from build123d import *

# Parameters (mm, degrees)
F0_W     = 130
F0_H     = 48
F1_DEPTH = 25
F3_DEPTH = 25.001
F4_R     = 1.5
F5_DEPTH = 25.001
F6_W     = 90
F6_H     = 48
F7_DEPTH = 5
F8_DEPTH = 25


with BuildPart() as f1:
    # F0 (on Top) → F1 (new body)
    with BuildSketch(Plane.XY):
        Rectangle(F0_W, F0_H)
    extrude(amount=F1_DEPTH)

    # F2 (on face) → F3 (cut, through all)
    with BuildSketch(Plane.XY.offset(25)):
        Polygon((7, -24), (0, -17), (-7, -24), align=None)
    extrude(amount=-F3_DEPTH, mode=Mode.SUBTRACT)

    # F4 (on face) → F5 (cut, through all)
    with BuildSketch(Plane.XY.offset(25)):
        with Locations((-55, 12)):
            Circle(F4_R)
        with Locations((-55, 2)):
            Circle(F4_R)
        with Locations((-55, -8)):
            Circle(F4_R)
        with Locations((55, 12)):
            Circle(F4_R)
        with Locations((55, 2)):
            Circle(F4_R)
        with Locations((55, -8)):
            Circle(F4_R)
    extrude(amount=-F5_DEPTH, mode=Mode.SUBTRACT)

    # F6 (on face) → F7 (join)
    with BuildSketch(Plane(origin=(0, 0, 0), x_dir=(1, 0, 0), z_dir=(0, 0, -1))):
        Rectangle(F6_W, F6_H)
    extrude(amount=F7_DEPTH)

    # F8 (cut): a face of the model
    f8_faces = [f1.faces().sort_by_distance(p)[0] for p in [
        (0, -21.6666666667, 0),
    ]]
    extrude(f8_faces, amount=-F8_DEPTH, mode=Mode.SUBTRACT)


solid = f1.part
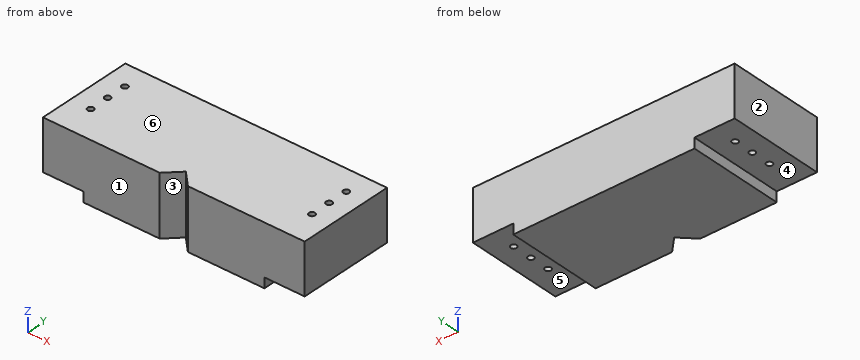
Part model, mm, in its own coordinate system. Face numbers are marked on the shaded views. A direction names the side the tool comes from. Coordinates: 2 decimals unless noted, no trailing zeros. Loops run counter-clockwise (first coordinate to the right, second up) from the corner with the lowest first, then second, coordinate; pieces in that order, holes last. Notation, with made-up numbers: (62, 18.5) -> (108, 18.5) arc R13 cw to (108, 35.5) -> close; hole circle Ø3 at (61, 11.25). An arc over 180 degrees is marked (long way). Use a Markdown table: item, result. Add a question column.
Item 1: Pull direction X, two halves, no side cores. Call the marked faces 1, 2 and 3: +X half, -X half, draft (parallel to the pull), parting line (faces both ways), or undercut.
Item 2: Band-saw the part on A-A on x = 55. Write the cut outline in (y, z), plus the area to 3 significant figures.
Item 3: Probe probe 1 along Y at (x, z) = (-55, 10.25); probe 2 along X at (y, z) = (2.5, 22); probe 3 along Z at (x, y) = (49.5, -16). List the from-to ranges inside material, lowest first.
Item 4: Which spindle directions (+Z, -Z, +X, -X, +Y, -Y) get a long thin tool onto all of the face, cutting with end or side? Do the marked faces 4, 5 and 6. Say none if no direction does.
Item 5: Band-saw the part on B-B on y = 12. Write the cut outline in (x, z), plus the area to 3 significant figures.
Item 6: Band-saw the part on D-D on x = -3. Write the cut outline in (y, z), plus the area to 3 significant figures.
Item 7: Flat gauge pins, fed straight in: P1, Ø1.5, axis at y = 10, z = -1.5, coming from the +X side; P2, Ø6, axis at x = -54, y = -5.5, coming from the -Z side; P3, Ø2.5, axis at x = 55, y = 2, coming from the -Z side; P4, Ø2.5, axis at y = 9, z = -2, coming from the -X side. Where does each tip first touch, or does it go through?
Item 8: Band-saw the part on C-C on y = -4.5. Write the cut outline in (x, z).
Geometry says:
| question | item | result |
|---|---|---|
| 1 | face 1 | draft |
| 1 | face 2 | -X half |
| 1 | face 3 | undercut |
| 2 | outline | (-24, 0) -> (-9.5, 0) -> (-9.5, 25) -> (-24, 25) -> close; (-6.5, 0) -> (0.5, 0) -> (0.5, 25) -> (-6.5, 25) -> close; (3.5, 0) -> (10.5, 0) -> (10.5, 25) -> (3.5, 25) -> close; (13.5, 0) -> (24, 0) -> (24, 25) -> (13.5, 25) -> close |
| 2 | area | 975 mm² |
| 3 | probe 1 | -24 to -9.5, -6.5 to 0.5, 3.5 to 10.5, 13.5 to 24 |
| 3 | probe 2 | -65 to -56.41, -53.59 to 53.59, 56.41 to 65 |
| 3 | probe 3 | 0 to 25 |
| 4 | face 4 | -Z, -X, +Y, -Y |
| 4 | face 5 | -Z, +X, +Y, -Y |
| 4 | face 6 | +Z, +X, -X, +Y, -Y |
| 5 | outline | (-65, 0) -> (-56.5, 0) -> (-56.5, 25) -> (-65, 25) -> close; (-53.5, 0) -> (-45, 0) -> (-45, -5) -> (45, -5) -> (45, 0) -> (53.5, 0) -> (53.5, 25) -> (-53.5, 25) -> close; (56.5, 0) -> (65, 0) -> (65, 25) -> (56.5, 25) -> close |
| 5 | area | 3,550 mm² |
| 6 | outline | (-20, -5) -> (24, -5) -> (24, 25) -> (-20, 25) -> close |
| 6 | area | 1,320 mm² |
| 7 | P1 | x = 45 |
| 7 | P2 | z = 0 |
| 7 | P3 | through |
| 7 | P4 | x = -45 |
| 8 | outline | (-65, 0) -> (-45, 0) -> (-45, -5) -> (45, -5) -> (45, 0) -> (65, 0) -> (65, 25) -> (-65, 25) -> close |
